```python
from build123d import *

# Parameters (mm, degrees)
SKETCH_1_R          = 6
EXTRUDE_4_DEPTH     = 18
FILLET_1_R          = 0.6
FILLET_6_R          = 0.7
EXTRUDE_5_DEPTH     = 9
SKETCH_3_R          = 2.55
CUT_EXTRUDE_1_DEPTH = 6
CHAMFER_1_SIZE      = 0.5
FILLET_4_R          = 0.5
FILLET_5_R          = 0.5
SKETCH_4_W          = 6.329239392
SKETCH_4_H          = 4.6
EXTRUDE_6_DEPTH     = 3.45
SKETCH_5_R          = 1.2
CUT_EXTRUDE_2_DEPTH = 3.45
CUT_EXTRUDE_START   = -13
SKETCH_7_R          = 6
SKETCH_7_R_2        = 5
CUT_EXTRUDE_4_DEPTH = 13
CHAMFER_2_SIZE      = 0.5


with BuildPart() as part:
    # ｽｹｯﾁ1 → ﾎﾞｽ - 押し出し4 (new body)
    with BuildSketch(Plane(origin=(0, 0, 0), x_dir=(1, 0, 0), z_dir=(0, 1, 0))):
        with Locations(Location((0, 0, 0), (0, 0, 270))):
            Circle(SKETCH_1_R)
        Polygon((-2.55, -0.95), (-2.55, 0.95), (-0.95, 0.95), (-0.95, 2.55), (0.95, 2.55), (0.95, 0.95), (2.55, 0.95), (2.55, -0.95), (0.95, -0.95), (0.95, -2.55), (-0.95, -2.55), (-0.95, -0.95), align=None, mode=Mode.SUBTRACT)
    extrude(amount=EXTRUDE_4_DEPTH)

    # ﾌｨﾚｯﾄ1
    fillet_1_edges = [part.edges().sort_by_distance(p)[0] for p in [
        (0.95, 9, -0.95),
    ]]
    fillet(fillet_1_edges, radius=FILLET_1_R)

    # ﾌｨﾚｯﾄ6
    fillet_6_edges = [part.edges().sort_by_distance(p)[0] for p in [
        (-0.95, 9, -0.95),
        (-0.95, 9, 0.95),
        (0.95, 9, 0.95),
    ]]
    fillet(fillet_6_edges, radius=FILLET_6_R)

    # ｽｹｯﾁ2 → ﾎﾞｽ - 押し出し5 (add)
    with BuildSketch(Plane.XZ):
        Polygon((6.92820323, 0), (3.464101615, 6), (-3.464101615, 6), (-6.92820323, 0), (-3.464101615, -6), (3.464101615, -6), align=None)
    extrude(amount=EXTRUDE_5_DEPTH)

    # ｽｹｯﾁ3 → ｶｯﾄ - 押し出し1 (cut)
    with BuildSketch(Plane.XZ.offset(9)):
        with Locations(Location((0, 0, 0), (0, 0, 270))):
            Circle(SKETCH_3_R)
    extrude(amount=-CUT_EXTRUDE_1_DEPTH, mode=Mode.SUBTRACT)

    # 面取り1
    chamfer_1_edges = [part.edges().sort_by_distance(p)[0] for p in [
        (0, -9, 2.55),
        (5.196152423, -9, -3),
        (5.196152423, -9, 3),
        (0, -9, 6),
        (-5.196152423, -9, 3),
        (-5.196152423, -9, -3),
        (0, -9, -6),
    ]]
    chamfer(chamfer_1_edges, length=CHAMFER_1_SIZE)

    # ﾌｨﾚｯﾄ4
    fillet_4_edges = [part.edges().sort_by_distance(p)[0] for p in [
        (-3.464101615, -4.25, 6),
    ]]
    fillet(fillet_4_edges, radius=FILLET_4_R)

    # ﾌｨﾚｯﾄ5
    fillet_5_edges = [part.edges().sort_by_distance(p)[0] for p in [
        (3.464101615, -4.25, -6),
        (-3.464101615, -4.25, -6),
        (-6.92820323, -4.25, 0),
        (3.464101615, -4.25, 6),
        (6.92820323, -4.25, 0),
    ]]
    fillet(fillet_5_edges, radius=FILLET_5_R)

    # ｽｹｯﾁ4 → ﾎﾞｽ - 押し出し6 (add)
    with BuildSketch(Plane.XY.offset(-2.55)):
        with Locations((0.010806785, 2.3)):
            Rectangle(SKETCH_4_W, SKETCH_4_H)
    extrude(amount=-EXTRUDE_6_DEPTH)

    # ｽｹｯﾁ5 → ｶｯﾄ - 押し出し2 (cut)
    with BuildSketch(Plane(origin=(0, 0, -6), x_dir=(-1, 0, 0), z_dir=(0, 0, -1))):
        with Locations((0, 2)):
            Circle(SKETCH_5_R)
    extrude(amount=-CUT_EXTRUDE_2_DEPTH, mode=Mode.SUBTRACT)

    # ｽｹｯﾁ7 → ｶｯﾄ - 押し出し4 (cut)
    with BuildSketch(Plane(origin=(0, 18, 0), x_dir=(1, 0, 0), z_dir=(0, 1, 0)).offset(CUT_EXTRUDE_START)):
        with Locations(Location((0, 0, 0), (0, 0, 270))):
            Circle(SKETCH_7_R)
        with Locations(Location((0, 0, 0), (0, 0, 270))):
            Circle(SKETCH_7_R_2, mode=Mode.SUBTRACT)
    extrude(amount=CUT_EXTRUDE_4_DEPTH, mode=Mode.SUBTRACT)

    # 面取り2
    chamfer_2_edges = [part.edges().sort_by_distance(p)[0] for p in [
        (0, 18, -5),
        (2.55, 18, 0),
        (-2.1, 18, -0.95),
        (-2.1, 18, 0.95),
        (-2.55, 18, 0),
        (2.05, 18, -0.95),
        (1.125735931, 18, -1.125735931),
        (-0.95, 18, 2.1),
        (2.1, 18, 0.95),
        (0.95, 18, 2.1),
        (1.155025253, 18, 1.155025253),
        (-1.155025253, 18, -1.155025253),
        (-1.155025253, 18, 1.155025253),
        (0.95, 18, -2.05),
        (0, 18, -2.55),
        (0, 18, 2.55),
        (-0.95, 18, -2.1),
    ]]
    chamfer(chamfer_2_edges, length=CHAMFER_2_SIZE)


solid = part.part
```
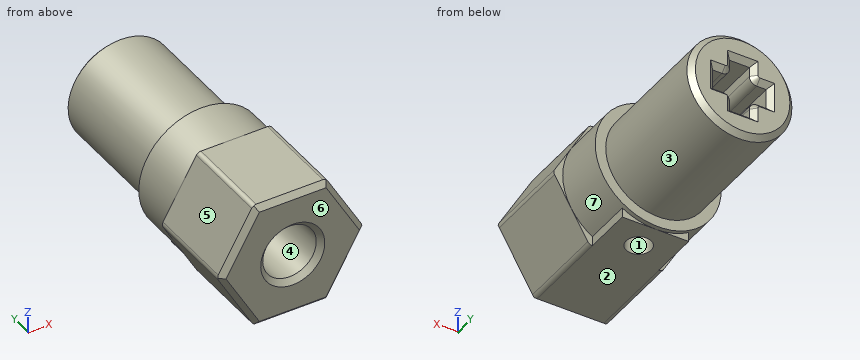
Can you work these out from the model? Positions are in its coordinate system, mm. Face numbers are marked on the shaded views. A direction names the side the tool comes from. Coordinates: 2 decimals unless noted, no trailing zeros. Loops run counter-clockwise (first coordinate to the right, second up) from the corner with the lowest first, then second, coordinate; pieces in that order, holes last. Notation, with made-up numbers: M 45.25,-11 L 87.25,-11 A26 cw 87.25,17 Z; hole C -22.75,49.25 d10. An arc over 180 degrees is marked long. Put each result on its own line as item: value. Start each with the question number.
(1) Imagine slicing it at A-A on y = 7. List the corners of the cut face in (x, z) for me.
(2) I need wall thicknesses on probe 1 along X at (y, z) = (-7.1, 0); probe 2 along Y at (x, z) = (0, -3.6); probe 3 along Z at (x, y) = (4, 7.25). Which ranges of each line are inside material? Lowest first, please.
(3) Will these pins go through, and if not, where does the flat tip stop? pin 1 Ø0.7 at (x, y) = (-2, 10) entering from -Z; pin 2 Ø2 at (x, z) = (4.5, 4.5) entering from +Y; pin 3 Ø5 at (y, z) = (13.5, 3) entering from +X.
(4) Imagine slicing it at C-C on y = -5.5. List the corners of the cut face in (x, z) for me.
(5) Which directions (+Z, -Z, +X, -X, +Y, -Y) give clear straight access to the entire face, cutting with the end or side of a thin tool? Please do the marked faces 1, 2 and 3.
(6) Imagine slicing it at B-B on y = 2. List the corners of the cut face in (x, z) for me, and give its area (3 significant figures).
(7) We'd pull the mould along X, two halves only. Please class the marked faces 4, 5, 6 and 7: +X half, -X half, draft (parallel to the pull), parting line (faces both ways), or undercut.
Worked answers:
1. outline: C 0,0 d10; hole M -2.55,-0.95 L -1.65,-0.95 A0.7 cw -0.95,-1.65 L -0.95,-2.55 L 0.95,-2.55 L 0.95,-1.55 A0.6 cw 1.55,-0.95 L 2.55,-0.95 L 2.55,0.95 L 1.65,0.95 A0.7 cw 0.95,1.65 L 0.95,2.55 L -0.95,2.55 L -0.95,1.65 A0.7 cw -1.65,0.95 L -2.55,0.95 Z
2. probe 1: x = -6.85 to -2.55, 2.55 to 6.85
2. probe 2: y = -9 to 0.8, 3.2 to 18
2. probe 3: z = -3 to 3
3. pin 1: stops at z = -4.72
3. pin 2: stops at y = 5
3. pin 3: stops at x = 4.97
4. outline: M -6.78,-0.25 L -3.61,-5.75 A0.5 ccw -3.18,-6 L 3.18,-6 A0.5 ccw 3.61,-5.75 L 6.78,-0.25 A0.5 ccw 6.78,0.25 L 3.61,5.75 A0.5 ccw 3.18,6 L -3.18,6 A0.5 ccw -3.61,5.75 L -6.78,0.25 A0.5 ccw Z; hole C 0,0 d5.1
5. face 1: -Z
5. face 2: -Z, +X, -X, +Y, -Y
5. face 3: +Y
6. outline: M -3.15,-6 L -1.2,-6 L -1.2,-2.55 L -0.95,-2.55 L -0.95,-1.65 A0.7 ccw -1.65,-0.95 L -2.55,-0.95 L -2.55,0.95 L -1.65,0.95 A0.7 ccw -0.95,1.65 L -0.95,2.55 L 0.95,2.55 L 0.95,1.65 A0.7 ccw 1.65,0.95 L 2.55,0.95 L 2.55,-0.95 L 1.55,-0.95 A0.6 ccw 0.95,-1.55 L 0.95,-2.55 L 1.2,-2.55 L 1.2,-6 L 3.18,-6 L 3.18,-5.09 A6 ccw long -3.15,-5.1 Z
6. area: 90.5 mm2
7. face 4: undercut
7. face 5: -X half
7. face 6: draft
7. face 7: parting line
